from build123d import *

# Parameters (mm, degrees)
F0_R     = 11
F0_R_2   = 5.5
F1_DEPTH = 2.5
F0_R_3   = 4.075
F2_DEPTH = 3
F3_DEPTH = 5.5
F4_R     = 1.5


with BuildPart() as f1:
    # F0 (on Front) → F1 (new body)
    with BuildSketch(Plane.XZ):
        Circle(F0_R)
        Circle(F0_R_2, mode=Mode.SUBTRACT)
    extrude(amount=F1_DEPTH)

    # F0 (on Front) → F2 (join)
    with BuildSketch(Plane.XZ):
        Circle(F0_R_2)
        Circle(F0_R_3, mode=Mode.SUBTRACT)
    extrude(amount=F2_DEPTH)

    # F0 (on Front) → F3 (join)
    with BuildSketch(Plane.XZ):
        Circle(F0_R_3)
    extrude(amount=F3_DEPTH)

    # F4
    f4_edges = [f1.edges().sort_by_distance(p)[0] for p in [
        (-11, 0, 0),
    ]]
    fillet(f4_edges, radius=F4_R)


solid = f1.part
Work out the finished part from the listing and answer in its coordinate system (mm). A direction names the side the tool comes from. Give positions to 0.01 mm unless a question says otherwise; leave off trailing zeros. Loops run counter-clockwise (first coordinate to the right, second up) from the corner with the lowest first, then second, coordinate; pieces in that order, holes last. Notation, with made-up numbers: (40, 54) - (56, 54) arc R6 ccw to (56, 65) - close; hole circle Ø9 at (-27, 32). An arc over 180 degrees is marked (long way). Answer in a Markdown table with one row per item. Add a question column.
Q1. A tool of negligible diameter and unlimited length cuts with its end or side. For faces 1 (the cylindrical face through (-2.38, -1.99, -10.74)), 2 (the flat face through (-4, -3, -2)), from which of +Z, -Z, +X, -X, +Y, -Y can it reach the whole face along a straight path? Write none if from no direction.
Q2. Consider line 1 along Y through (x, z) = (1.75, -8.5); line 2 along X through (y, z) = (-1.65, 5.25); line 3 along Z through (x, y) = (8.25, -2.4). Determine where each line is inside the solid, lowest interval first.
Q3. The part is cut by section B-B (x = 0). Determine the outline of the cut face in (y, z) (3 decimals), and give its area (3 significant figures).
Q4. Determine the mould class of faces 3 (the flat face through (-3, -2.5, 5)), 4 (the flat face through (0, 0, 0)), 5 (the cylindrical face through (-1.19, -2.75, -5.37)) for opening direction Y: released by +Y, released by -Y, zero draft, split by the parting line, or undercut.
Q5. Each of these flat-tipped pins is pushed along its axis until it touches: P1, Ø1.5, axis at y = -3, z = 7, coming from the +X side; P2, Ø3, axis at x = -2.5, y = -3, coming from the +Z side; P3, Ø1, axis at x = 3, z = -3.5, coming from the -Y side. Where does it stop, or does it pass through?
Q6. The part is cut by section A-A (z = 0). Determine the outline of the cut face in (x, y) (3 decimals).
Q7. The part is cut by section D-D (y = -0.7). Determine the outline of the cut face in (x, z).
Q8. The part is cut by section C-C (y = -3.35). Determine the outline of the cut face in (x, z) (3 decimals), and give its area (3 significant figures).
Solution:
| question | item | result |
|---|---|---|
| 1 | face 1 | +Y, -Y |
| 1 | face 2 | -Y |
| 2 | line 1 | y = -2.5 to 0 |
| 2 | line 2 | x = -9.67 to 9.67 |
| 2 | line 3 | z = -7.28 to 7.28 |
| 3 | outline | (-5.5, -4.075) - (-3, -4.075) - (-3, -5.5) - (-2.5, -5.5) - (-2.5, -11) - (-1.5, -11) arc R1.5 ccw to (0, -9.5) - (0, 9.5) arc R1.5 ccw to (-1.5, 11) - (-2.5, 11) - (-2.5, 5.5) - (-3, 5.5) - (-3, 4.075) - (-5.5, 4.075) - close |
| 3 | area | 79.9 mm² |
| 4 | face 3 | released by -Y |
| 4 | face 4 | released by +Y |
| 4 | face 5 | zero draft |
| 5 | P1 | stops at x = 8.92 |
| 5 | P2 | stops at z = 10.95 |
| 5 | P3 | stops at y = -3 |
| 6 | outline | (-11, -2.5) - (-5.5, -2.5) - (-5.5, -3) - (-4.075, -3) - (-4.075, -5.5) - (4.075, -5.5) - (4.075, -3) - (5.5, -3) - (5.5, -2.5) - (11, -2.5) - (11, -1.5) arc R1.5 ccw to (9.5, 0) - (-9.5, 0) arc R1.5 ccw to (-11, -1.5) - close |
| 7 | outline | circle Ø21.54 at (0, 0) |
| 8 | outline | circle Ø8.15 at (0, 0) |
| 8 | area | 52.2 mm² |
